Job drawing, mm, ordinate dimensions from the low corner. One solid piece. A direction names the side the tool comes from. Round coordinates to 2 decimals unless told otherwise and drop trailing zeros. Loops run counter-clockwise (first coordinate to the right, second up) from the corner with the lowest first, then second, coordinate; pieces in that order, holes last. Notation, with made-up numbers: M -15,64 L -7,64 A13 cw -7,70 Z; hole C 33,51 d5. An arc over 180 degrees is marked long. One line per item, written item: value.
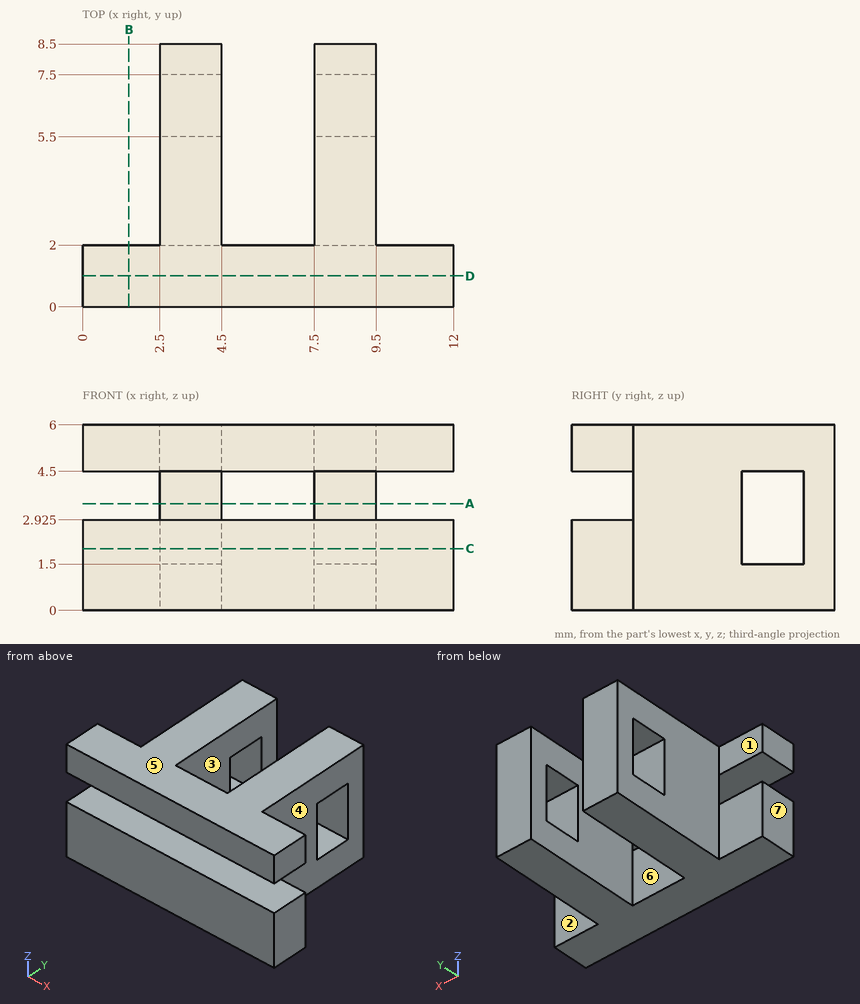
Item 1: Slice it at C-C, the plane z = 2. Give the cut face in (x, y), and give its area (3 significant figures).
Check values:
outline: M 0,0 L 12,0 L 12,2 L 9.5,2 L 9.5,5.5 L 7.5,5.5 L 7.5,2 L 4.5,2 L 4.5,5.5 L 2.5,5.5 L 2.5,2 L 0,2 Z; M 2.5,7.5 L 4.5,7.5 L 4.5,8.5 L 2.5,8.5 Z; M 7.5,7.5 L 9.5,7.5 L 9.5,8.5 L 7.5,8.5 Z
area: 42.0 mm2
Item 2: Drop flat-ended pins along their axis: P1, Ø1.2, axis at x = 6, z = 5, coming from the +Y side; P2, Ø0.8, axis at x = 4, z = 3.5, coming from the -Y side; P3, Ø3, axis at y = 5, z = 2.5, coming from the +X side; P4, Ø1.5, axis at x = 6, y = 4, coming from the -Z side. Give the stop position or say it passes through.
Check values:
P1: stops at y = 2
P2: stops at y = 2
P3: stops at x = 9.5
P4: passes through
Item 3: Slice it at D-D, the plane y = 1. Give the cut face in (x, z) (1 decimal), and give its area (3 significant figures).
Check values:
outline: M 0,0 L 12,0 L 12,2.9 L 0,2.9 Z; M 0,4.5 L 12,4.5 L 12,6 L 0,6 Z
area: 53.1 mm2
Item 4: Slice it at A-A, the plane z = 3.45. Give the cut face in (x, y).
Check values:
outline: M 2.5,2 L 4.5,2 L 4.5,5.5 L 2.5,5.5 Z; M 2.5,7.5 L 4.5,7.5 L 4.5,8.5 L 2.5,8.5 Z; M 7.5,2 L 9.5,2 L 9.5,5.5 L 7.5,5.5 Z; M 7.5,7.5 L 9.5,7.5 L 9.5,8.5 L 7.5,8.5 Z
Item 5: Pull direction X, two halves, no side cores. Call the marked faces 4, 5, 6 and 7: pulls with the +X half, pulls with the -X half, needs draft (parallel to the pull), parting line crosses it, or undercut.
Check values:
face 4: pulls with the +X half
face 5: needs draft
face 6: undercut
face 7: pulls with the -X half
Item 6: Wall check: line 1 along X through (y, z) = (3.5, 3.9); line 2 along Z through (x, y) = (6.5, 0.5) (1 decimal); line 3 along Y through (x, z) = (1, 2.15). Give the ranges that are in metal, low to high.
Check values:
line 1: x = 2.5 to 4.5, 7.5 to 9.5
line 2: z = 0 to 2.9, 4.5 to 6
line 3: y = 0 to 2
Item 7: Slice it at B-B, the plane x = 1.5. Give the cut face in (y, z) (1 decimal).
Check values:
outline: M 0,0 L 2,0 L 2,2.9 L 0,2.9 Z; M 0,4.5 L 2,4.5 L 2,6 L 0,6 Z
Item 8: Which spindle directions (+Z, -Z, +X, -X, +Y, -Y) get a long thin tool onto all of the face, cutting with end or side? Do the marked faces 1, 2 and 3. Say none if no direction does.
Check values:
face 1: +Z, -Z, -X, +Y
face 2: +Z, -Z, +X, +Y
face 3: +Z, -Z, +Y
